from build123d import *

# Parameters (mm, degrees)
SKETCH_1_W          = 24
SKETCH_1_H          = 70
EXTRUDE_1_DEPTH     = 30
SKETCH_2_R          = 7.55
CUT_EXTRUDE_1_DEPTH = 71.806439045
SKETCH_3_W          = 25
SKETCH_3_H          = 10
CUT_EXTRUDE_2_DEPTH = 71.806439045
FILLET_1_R          = 10
SKETCH_6_W          = 24
SKETCH_6_H          = 7.198600856
EXTRUDE_3_DEPTH     = 15
EXTRUDE_4_DEPTH     = 24
EXTRUDE_5_DEPTH     = 8
EXTRUDE_6_DEPTH     = 8
SKETCH_10_R         = 15
CUT_EXTRUDE_4_DEPTH = 16
EXTRUDE_7_DEPTH     = 7.198600855
EXTRUDE_8_DEPTH     = 7.198600855
FILLET_2_R          = 10
FILLET_3_R          = 10
SKETCH_14_R         = 3.499999999
CUT_EXTRUDE_5_DEPTH = 13
SKETCH_16_R         = 1.599999999
SKETCH_16_R_2       = 1.550452657
CUT_EXTRUDE_6_DEPTH = 26


with BuildPart() as part:
    # 草图1 → 凸台-拉伸1 (new body)
    with BuildSketch(Plane(origin=(0, 0, 0), x_dir=(1, 0, 0), z_dir=(0, 1, 0))):
        with Locations((20.241900648, -24.477321814)):
            Rectangle(SKETCH_1_W, SKETCH_1_H)
    extrude(amount=EXTRUDE_1_DEPTH)

    # 草图2 → 切除-拉伸1 (cut, through all)
    with BuildSketch(Plane(origin=(32.241900648, 0, 0), x_dir=(0, 0, -1), z_dir=(1, 0, 0))):
        with Locations((-46.977321814, 15)):
            Circle(SKETCH_2_R)
        with Locations((-1.977321814, 15)):
            Circle(SKETCH_2_R)
    extrude(amount=-CUT_EXTRUDE_1_DEPTH, mode=Mode.SUBTRACT)

    # 草图3 → 切除-拉伸2 (cut, through all)
    with BuildSketch(Plane(origin=(32.241900648, 0, 0), x_dir=(0, 0, -1), z_dir=(1, 0, 0))):
        with Locations((-24.477321814, 15)):
            Rectangle(SKETCH_3_W, SKETCH_3_H)
    extrude(amount=-CUT_EXTRUDE_2_DEPTH, mode=Mode.SUBTRACT)

    # 圆角1
    fillet_1_edges = [part.edges().sort_by_distance(p)[0] for p in [
        (20.241900648, 30, -10.522678186),
        (20.241900648, 0, -10.522678186),
        (20.241900648, 0, 59.477321814),
        (20.241900648, 30, 59.477321814),
    ]]
    fillet(fillet_1_edges, radius=FILLET_1_R)

    # 草图6 → 凸台-拉伸3 (add)
    with BuildSketch(Plane(origin=(0, 30, 0), x_dir=(1, 0, 0), z_dir=(0, 1, 0))):
        with Locations((20.241900648, -38.481509693)):
            Rectangle(SKETCH_6_W, SKETCH_6_H)
    extrude(amount=EXTRUDE_3_DEPTH)

    # 草图7 → 凸台-拉伸4 (add)
    with BuildSketch(Plane.ZY.offset(-8.241900648)):
        Polygon((42.080810121, 45), (21.912574503, 79.54333904), (15.694773475, 75.913056629), (34.882209265, 45), align=None)
    extrude(amount=-EXTRUDE_4_DEPTH)

    # 草图8 → 凸台-拉伸5 (add)
    with BuildSketch(Plane.ZY.offset(-8.241900648)):
        Polygon((42.080810121, 45), (34.882209265, 45), (15.694773475, 75.913056629), (21.912574503, 79.54333904), align=None)
    extrude(amount=EXTRUDE_5_DEPTH)

    # 草图9 → 凸台-拉伸6 (add)
    with BuildSketch(Plane(origin=(32.241900648, 0, 0), x_dir=(0, 0, -1), z_dir=(1, 0, 0))):
        Polygon((-42.080810121, 45), (-34.882209265, 45), (-15.694773475, 75.913056629), (-21.912574503, 79.54333904), align=None)
    extrude(amount=EXTRUDE_6_DEPTH)

    # 草图10 → 切除-拉伸4 (cut)
    with BuildSketch(Plane(origin=(0, 29.763050525, 50.976950321), x_dir=(1, 0, 0), z_dir=(0, 0.5042058904481267, 0.8635834760099408))):
        with Locations(Location((20.241900648, 37.643864083, 0), (0, 0, 270))):
            Circle(SKETCH_10_R)
    extrude(amount=-CUT_EXTRUDE_4_DEPTH, mode=Mode.SUBTRACT)

    # 草图12 → 凸台-拉伸7 (add)
    with BuildSketch(Plane.XY.offset(42.080810121)):
        Polygon((0.241900648, 45), (8.241900648, 45), (8.241900648, 30), align=None)
    extrude(amount=-EXTRUDE_7_DEPTH)

    # 草图13 → 凸台-拉伸8 (add)
    with BuildSketch(Plane.XY.offset(42.080810121)):
        Polygon((40.241900648, 45), (32.241900648, 45), (32.241900648, 30), align=None)
    extrude(amount=-EXTRUDE_8_DEPTH)

    # 圆角2
    fillet_2_edges = [part.edges().sort_by_distance(p)[0] for p in [
        (20.241900648, 45, 42.080810121),
    ]]
    fillet(fillet_2_edges, radius=FILLET_2_R)

    # 圆角3
    fillet_3_edges = [part.edges().sort_by_distance(p)[0] for p in [
        (0.241900648, 45, 38.295029227),
        (40.241900648, 45, 38.295029227),
    ]]
    fillet(fillet_3_edges, radius=FILLET_3_R)

    # 草图14 → 切除-拉伸5 (cut)
    with BuildSketch(Plane.XY.offset(42.080810121)):
        with Locations((20.170389916, 36.617139635)):
            Circle(SKETCH_14_R)
    extrude(amount=-CUT_EXTRUDE_5_DEPTH, mode=Mode.SUBTRACT)

    # 草图16 → 切除-拉伸6 (cut)
    with BuildSketch(Plane(origin=(0, 30, 0), x_dir=(1, 0, 0), z_dir=(0, 1, 0))):
        with Locations(Location((13.070026875, -15.228876714, 0), (0, 0, 270))):
            Circle(SKETCH_16_R)
        with Locations(Location((27.370026875, -15.228876714, 0), (0, 0, 270))):
            Circle(SKETCH_16_R_2)
    extrude(amount=-CUT_EXTRUDE_6_DEPTH, mode=Mode.SUBTRACT)


solid = part.part
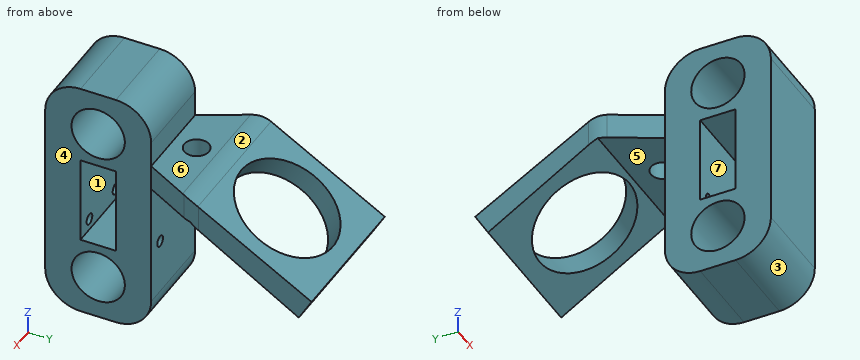
Source: CAD feature listing. Evaluate the final solid. Frame: model axes, mm. Face numbers are marked on the shaded views. A direction names the side the tool comes from. Give positions to 0.01 mm unless a question says otherwise; leave off trailing zeros. Write each loop counter-clockwise with the first axis right and the second up, starting at its lowest first coordinate (ties: lowest second). Pieces come first, ordered by that corner, then holes. Notation, with made-up numbers: (84.25, 2.25) -> (126.25, 2.25) arc R31 ccw to (126.25, 31.25) -> close; hole circle Ø6 at (-24, 57.25). An arc over 180 degrees is marked (long way). Write item = value, one per line.
Q1. Mould query, pull axis Y, two halves, no side actions, for the marked faces 1, 2 and 3. Classes: +Y half, -Y half, draft (parallel to the pull), parting line (faces both ways), or undercut.
Here are the results:
face_1 = undercut
face_2 = +Y half
face_3 = -Y half
Q2. Cut plane C-C on z = 44. Return loops of the section in (x, y).
Here are the results:
outline = (8.24, 0) -> (32.24, 0) -> (32.24, 8.06) -> (8.24, 8.06) -> close; (8.24, 21.94) -> (32.24, 21.94) -> (32.24, 30) -> (8.24, 30) -> close
Q3. Cut plane D-D on x = 10. Return loops of the section in (y, z), then the cut area to 3 significant figures.
Here are the results:
outline = (0, -0.52) arc R10 ccw to (10, -10.52) -> (20, -10.52) arc R10 ccw to (30, -0.52) -> (30, 34.88) -> (45, 34.88) -> (49.6, 32.03) -> (52.81, 37.52) -> (47.34, 40.72) arc R10 ccw to (42.29, 42.08) -> (30, 42.08) -> (30, 49.48) arc R10 ccw to (20, 59.48) -> (10, 59.48) arc R10 ccw to (0, 49.48) -> close; (68.23, 20.46) -> (75.91, 15.69) -> (79.54, 21.91) -> (71.74, 26.47) -> close; hole circle Ø15.1 at (15, 1.98); hole circle Ø15.1 at (15, 46.98); hole (10, 11.98) -> (20, 11.98) -> (20, 36.98) -> (10, 36.98) -> close
area = 1,620 mm²
Q4. Reachability of the marked faces 4, 5, 6 and 7 from +Z, -Z, +X, -X, +Y, -Y: full face, straight path, thin tool, end or side. Return the list, or none.
Here are the results:
face_4 = +Z, -Z, +X, -Y
face_5 = -Z, +X, -X
face_6 = +Z, +X, -X, +Y
face_7 = +X, -X
Q5. Cut plane B-B on x = 22. State how many separate pieces and enclosed holes the cut face has, then the cut area to 3 significant figures.
Here are the results:
separate_pieces = 3
enclosed_holes = 3
area = 1,530 mm²
Q6. First-contact query: pin 1 (9 mm diameter, centred on y = 21.5, z = 17.5, fed in from -X); pin 2 (15 mm diameter, centred on y = 20.5, z = 9.5, fed in from +X); pin 3 (4.5 mm diameter, centred on x = 11, y = 36.5, fed in from -Z); pin 4 (3 mm diameter, centred on x = 34, y = 14.5, fed in from +Z). Flat tips, straight axial feed; report the tip coordinate or a pass-through.
Here are the results:
pin_1 = 8.24
pin_2 = 32.24
pin_3 = 34.88
pin_4 = through
Q7. Line query: line 1 (Z direction, x = 16.5, y = 9); line 2 (Y direction, x = 10, z = 29.5); line 3 (X direction, y = 27, z = 17). Output: solid intervals per line, ascending. Write a range as from..to.
Here are the results:
line_1 = -10.47..-2.61, 6.56..42.39, 51.56..59.43
line_2 = 0..10, 20..30
line_3 = 8.24..32.24
Q8. Cut plane A-A on y = 15. Return loops of the section in (x, z), then the cut area to 3 significant figures.
Here are the results:
outline = (8.24, -10.52) -> (32.24, -10.52) -> (32.24, -5.57) -> (8.24, -5.57) -> close; (8.24, 9.53) -> (32.24, 9.53) -> (32.24, 11.98) -> (8.24, 11.98) -> close; (8.24, 36.98) -> (32.24, 36.98) -> (32.24, 39.43) -> (8.24, 39.43) -> close; (8.24, 54.53) -> (32.24, 54.53) -> (32.24, 59.48) -> (8.24, 59.48) -> close
area = 355 mm²
